```python
from build123d import *

# Parameters (mm, degrees)
SKETCH2_R               = 20
BOSS_EXTRUDE2_DEPTH     = 50
CUT_EXTRUDE1_DEPTH      = 20
FILLET1_R               = 12.5
CUT_EXTRUDE2_DEPTH      = 61.466933273
CUT_EXTRUDE2_DEPTH_BACK = 61.466933273
SKETCH4_R               = 4
SKETCH5_R               = 40
BOSS_EXTRUDE3_DEPTH     = 65
SKETCH7_R               = 4
BOSS_EXTRUDE5_DEPTH     = 30
CIRPATTERN1_COUNT       = 3
SKETCH8_W               = 90
SKETCH8_H               = 100
BOSS_EXTRUDE6_DEPTH     = 90
SKETCH9_R               = 35
BOSS_EXTRUDE7_DEPTH     = 70


with BuildPart() as part:
    # Sketch2 → Boss-Extrude2 (new body)
    with BuildSketch(Plane(origin=(0, 0, 0), x_dir=(0, 0, -1), z_dir=(1, 0, 0))):
        Circle(SKETCH2_R)
    extrude(amount=BOSS_EXTRUDE2_DEPTH)

    # Sketch3 → Cut-Extrude1 (cut)
    with BuildSketch(Plane.ZY):
        with BuildLine():
            Line((-7.5, 18.540496218), (-7.5, -18.540496218))
            ThreePointArc((-7.5, -18.540496218), (0, -20), (7.5, -18.540496218))
            Line((7.5, -18.540496218), (7.5, 18.540496218))
            ThreePointArc((7.5, 18.540496218), (0, 20), (-7.5, 18.540496218))
        make_face()
    extrude(amount=-CUT_EXTRUDE1_DEPTH, mode=Mode.SUBTRACT)

    # Fillet1
    fillet1_edges = [part.edges().sort_by_distance(p)[0] for p in [
        (0, 0, 7.5),
        (0, 0, -7.5),
    ]]
    fillet(fillet1_edges, radius=FILLET1_R - 0.0001)  # a hair under: the kernel refuses the full size

    # Sketch4 → Cut-Extrude2 (cut, two sides: drawn at the far end of the back side and taken through both)
    with BuildSketch(Plane.XY.offset(-7.5).offset(-CUT_EXTRUDE2_DEPTH_BACK)):
        with Locations((10, 0)):
            Circle(SKETCH4_R)
    extrude(amount=CUT_EXTRUDE2_DEPTH + CUT_EXTRUDE2_DEPTH_BACK, mode=Mode.SUBTRACT)

    # Sketch5 → Boss-Extrude3 (add)
    with BuildSketch(Plane(origin=(50, 0, 0), x_dir=(0, 0, -1), z_dir=(1, 0, 0))):
        Circle(SKETCH5_R)
    extrude(amount=BOSS_EXTRUDE3_DEPTH)

    # Sketch7 → Boss-Extrude5 (add)
    with BuildSketch(Plane.ZY.offset(-50)):
        with Locations(Location((0, 32, 0), (0, 0, 180))):
            Circle(SKETCH7_R)
    boss_extrude5 = extrude(amount=BOSS_EXTRUDE5_DEPTH)

    # CirPattern1: Boss-Extrude5 ×3 about axis
    cirpattern1_axis = Axis((0, 0, 0), (1, 0, 0))
    for i in range(1, CIRPATTERN1_COUNT):
        add(boss_extrude5.rotate(cirpattern1_axis, i * 360 / CIRPATTERN1_COUNT))

    # Sketch8 → Boss-Extrude6 (add)
    with BuildSketch(Plane(origin=(115, 0, 0), x_dir=(0, 0, -1), z_dir=(1, 0, 0))):
        with Locations((0, 5)):
            Rectangle(SKETCH8_W, SKETCH8_H)
    extrude(amount=BOSS_EXTRUDE6_DEPTH)

    # Sketch9 → Boss-Extrude7 (add)
    with BuildSketch(Plane(origin=(0, 55, 0), x_dir=(1, 0, 0), z_dir=(0, 1, 0))):
        with Locations(Location((160, 0, 0), (0, 0, 90))):
            Circle(SKETCH9_R)
    extrude(amount=BOSS_EXTRUDE7_DEPTH)


solid = part.part
```
Work out the finished part from the listing and answer in its coordinate system (mm). A direction names the side the tool comes from. Give positions to 0.01 mm unless a question says otherwise; leave off trailing zeros. Order: outer loops, then holes, each group sorted by start corner. A loop starts at its lowest first (then second) coordinate and runs counter-clockwise, first axis right, second up.
1. Section D-D, the plane x = 10 is taken. Determine the outline of the cut face in (y, z).
Result sheet:
outline: (-18.44, -7.75) arc R20 ccw to (-4, -19.6) - (-4, -7.75) - close; (-18.44, 7.75) - (-4, 7.75) - (-4, 19.6) arc R20 ccw to start; (4, -19.6) arc R20 ccw to (18.44, -7.75) - (4, -7.75) - close; (4, 7.75) - (18.44, 7.75) arc R20 ccw to (4, 19.6) - close
2. Section A-A, the plane z = 0 is taken. Determine the outline of the cut face in (x, y).
Result sheet:
outline: (20, -20) - (50, -20) - (50, -40) - (115, -40) - (115, -45) - (205, -45) - (205, 55) - (195, 55) - (195, 125) - (125, 125) - (125, 55) - (115, 55) - (115, 40) - (50, 40) - (50, 36) - (20, 36) - (20, 28) - (50, 28) - (50, 20) - (20, 20) - close
3. Each of these flat-tipped pins is pushed along its axis until it touches: P1, Ø2, axis at x = 45.5, z = 24, coming from the +Y side; P2, Ø2.5, axis at y = -17, z = -29.5, coming from the -X side; P3, Ø5, axis at y = 27, z = -5, coming from the -X side. Where does it stop, or does it pass through?
Result sheet:
P1: stops at y = -13.06
P2: stops at x = 20
P3: stops at x = 50
4. For faces 4 (the flat face through (20, -16, 28)), 5 (the cylindrical face through (35.21, -17.201, 23.898)), 6 (the cylindrical face through (3.564, -0.26, -11.259)), determine the directions among +Z, -Z, +X, -X, +Y, -Y from which every point of the face is accessible in a straight line to the end or side of a thin tool.
Result sheet:
face 4: +Z, -X, +Y, -Y
face 5: -X
face 6: -X, +Y, -Y
5. The mould has two halves that part along Z. Classify faces 1 (the flat face through (16, 0, 7.5)), 2 (the flat face through (159, 4, 45)), 3 (the cylindrical face through (194.168, 89.51, 7.587)): released by +Z, released by -Z, zero draft, split by the parting line, or undercut.
Result sheet:
face 1: undercut
face 2: released by +Z
face 3: split by the parting line
6. Straight lines are drawn through the part: L1, parallel to Y at x = 121.5, z = 36.5; L2, parallel to X at y = 0, z = -12; L3, parallel to Y at x = 10, z = 14.5. For each, find the intervals that lie inside material, in ascending order.
Result sheet:
L1: y = -45 to 55
L2: x = 2.9 to 6, 14 to 205
L3: y = -13.77 to -4, 4 to 13.77
7. Section B-B, the plane x = 160 is taken. Determine the outline of the cut face in (y, z), and give its area (3 significant figures).
Result sheet:
outline: (-45, -45) - (55, -45) - (55, -35) - (125, -35) - (125, 35) - (55, 35) - (55, 45) - (-45, 45) - close
area: 13,900 mm2
8. Section C-C, the plane y = 32 is taken. Determine the outline of the cut face in (x, z).
Result sheet:
outline: (20, -4) - (50, -4) - (50, -24) - (115, -24) - (115, -45) - (205, -45) - (205, 45) - (115, 45) - (115, 24) - (50, 24) - (50, 4) - (20, 4) - close
